Check sheet for the modelled part. Datum: model origin and axes. Units: mm. Face numbers are marked on the shaded views. A direction names the side the tool comes from. Give positions to 0.01 mm unless a question says otherwise; leave off trailing zeros. Write each loop counter-clockwise with the first axis right and the second up, starting at its lowest first coordinate (ties: lowest second). Pieces come first, ordered by that corner, then holes.
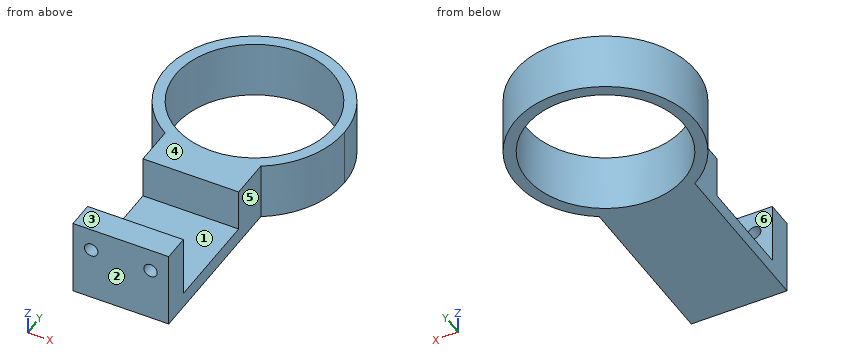
from build123d import *

# Parameters (mm, degrees)
F0_R     = 20.5
F1_DEPTH = 15
F0_W     = 25
F0_H     = 26.5
F2_DEPTH = 4
F0_H_2   = 7
F3_DEPTH = 20
F4_R     = 1.75
F5_DEPTH = 7


# Not quite as in the source:
# - a feature names something its author has since deleted; it is built from what else it names


with BuildPart() as f1:
    # F0 (on Top) → F1 (new body)
    with BuildSketch(Plane.XY):
        with BuildLine():
            ThreePointArc((12.5, -19.8997487421), (0, -23.5), (-12.5, -19.8997487421))
            Line((-12.5, -19.8997487421), (-12.5, -30.5))
            Line((-12.5, -30.5), (12.5, -30.5))
            Line((12.5, -30.5), (12.5, -19.8997487421))
        make_face()
        with BuildLine():
            ThreePointArc((23.5, 0), (-11.3688170009, 20.5669638012), (-12.5, -19.8997487421))
            ThreePointArc((-12.5, -19.8997487421), (0, -23.5), (12.5, -19.8997487421))
            ThreePointArc((12.5, -19.8997487421), (20.5669638012, -11.3688170009), (23.5, 0))
        make_face()
        Circle(F0_R, mode=Mode.SUBTRACT)
    extrude(amount=F1_DEPTH)

    # F0 (on Top) → F2 (join)
    with BuildSketch(Plane.XY):
        with BuildLine():
            ThreePointArc((12.5, -19.8997487421), (0, -23.5), (-12.5, -19.8997487421))
            Line((-12.5, -19.8997487421), (-12.5, -30.5))
            Line((-12.5, -30.5), (12.5, -30.5))
            Line((12.5, -30.5), (12.5, -19.8997487421))
        make_face()
        with Locations((0, -43.75)):
            Rectangle(F0_W, F0_H)
    extrude(amount=F2_DEPTH)

    # F0 (on Top) → F3 (join)
    with BuildSketch(Plane.XY):
        with Locations((0, -60.5)):
            Rectangle(F0_W, F0_H_2)
    extrude(amount=F3_DEPTH)

    # F4 (on face) → F5 (cut, through all)
    with BuildSketch(Plane.XZ.offset(64)):
        with Locations((-7.75, 14)):
            Circle(F4_R)
        with Locations((7.75, 14)):
            Circle(F4_R)
    extrude(amount=-F5_DEPTH, mode=Mode.SUBTRACT)


solid = f1.part
1) Gauge pin test, flat ends, axial feed: pin 1 (1 mm diameter, centred on x = 2, z = 9.5, fed in from +Y); pin 2 (3 mm diameter, centred on x = -7.75, z = 14, fed in from +Y); pin 3 (4 mm diameter, centred on y = -13, z = 13, fed in from -X); pin 4 (8 mm diameter, centred on x = -0.5, z = 9.5, fed in from +Y). Record the tip position at first contact, or that the pin passes through.
2) Access from +Z, -Z, +X, -X, +Y, -Y to the whole of each face (thin tool, end or side, straight path). Record for the marked faces 4, 5 and 6.
3) Sectioned sample at D-D on y = 15. Record the boundary of the cut face in (x, z), then the cut area to 3 significant figures.
4) Draft check along Y on the marked faces 1, 2 and 3. Enter one of: +Y half, -Y half, draft (parallel to the pull), parting line (faces both ways), or undercut.
5) Sectioned sample at A-A on z = 14. Record the boundary of the cut face in (x, y), then the cut area to 3 significant figures.
6) Scan lines: L1, parallel to Y at x = 0, z = 11.25; L2, parallel to Z at x = -7.75, y = -61.5; L3, parallel to Y at x = 10, z = 10.5. Record each from-to range of solid material in increasing order.
7) Sectioned sample at B-B on x = 0. Record the boundary of the cut face in (y, z).
8) Sectioned sample at C-C on z = 8. Record the boundary of the cut face in (x, y), then the cut area to 3 significant figures.
Answers below:
1. pin 1: stops at y = 23.45
1. pin 2: stops at y = 22.65
1. pin 3: stops at x = -20.77
1. pin 4: stops at y = 23.5
2. face 4: +Z, +X, -X, +Y
2. face 5: +Z, -Z, +X, -Y
2. face 6: +Z, +X, -X
3. outline: (-18.09, 0) - (-13.97, 0) - (-13.97, 15) - (-18.09, 15) - close; (13.97, 0) - (18.09, 0) - (18.09, 15) - (13.97, 15) - close
3. area: 124 mm2
4. face 1: undercut
4. face 2: -Y half
4. face 3: draft
5. outline: (-12.5, -64) - (-9.5, -64) - (-9.5, -57) - (-12.5, -57) - close; (-12.5, -30.5) - (12.5, -30.5) - (12.5, -19.9) arc R23.5 ccw (long way) to (-12.5, -19.9) - close; (-6, -64) - (6, -64) - (6, -57) - (-6, -57) - close; (9.5, -64) - (12.5, -64) - (12.5, -57) - (9.5, -57) - close; hole circle Ø41 at (0, 0)
5. area: 745 mm2
6. L1: y = -64 to -57, -30.5 to -20.5, 20.5 to 23.5
6. L2: z = 0 to 12.25, 15.75 to 20
6. L3: y = -64 to -57, -30.5 to -17.9, 17.9 to 21.27
7. outline: (-64, 0) - (-20.5, 0) - (-20.5, 15) - (-30.5, 15) - (-30.5, 4) - (-57, 4) - (-57, 20) - (-64, 20) - close; (20.5, 0) - (23.5, 0) - (23.5, 15) - (20.5, 15) - close
8. outline: (-12.5, -64) - (12.5, -64) - (12.5, -57) - (-12.5, -57) - close; (-12.5, -30.5) - (12.5, -30.5) - (12.5, -19.9) arc R23.5 ccw (long way) to (-12.5, -19.9) - close; hole circle Ø41 at (0, 0)
8. area: 794 mm2
